The model under review builds one solid part; all positions refer to its coordinate system, in mm. A direction names the side the tool comes from. Coordinates: 2 decimals unless noted, no trailing zeros. Write each loop counter-clockwise with the first axis right and the second up, starting at its lowest first coordinate (ties: lowest second). Pieces come first, ordered by that corner, then holes. Notation, with made-up numbers: (-33.75, -22) - (7.25, -22) arc R24 cw to (7.25, -4) - close; hole circle Ø11 at (77.25, 18.5). An arc over 180 degrees is marked (long way). Return JSON: item names as keys, results as strings. Group by question number.
(1) Tool access review of faces 4 (the face through (-1.74, 6.11, 0.76)), 5 (the face through (-3, 2, 1.016)), 6 (the face through (-2, -5, 0.508)), 7 (the face through (1.75, 6.14, 0.76)): name each direction out of +Z, -Z, +X, -X, +Y, -Y from which nothing blocks a thin tool from reaching the whole face with its end or side.
(2) We need section B-B on x = 0. State the section outline as (y, z) points, then the cut area to 3 significant figures.
(3) To check wall thickness, follow L1, parallel to Y at x = 0, z = 0.1; L2, parallel to Z at x = -2.5, y = 3.5; L3, parallel to Z at x = -2, y = 5.5. State the ranges of each line that lie inside material, in increasing order. Write a range as from..to.
(4) Draft analysis for pull direction X (two halves, no side actions). For faces 1 (the face through (0, -7, 3.734)), 2 (the face through (1.75, -6.14, 0.76)), 3 (the face through (-0.75, -3.39, 0.25)), state which applies: released by +X, released by -X, zero draft, split by the parting line, or undercut.
(5) For pin 1 Ø2 at (x, z) = (-3, 0.5) entering from +Y; pin 2 Ø1.4 at (x, z) = (0.5, 2.5) entering from +Y; pin 3 Ø0.9 at (y, z) = (-7, 3) entering from +X, all flat-tipped, find the tip position at first contact; note any pin that passes through.
(6) We need section A-A on y = 0. State the section outline as (x, z) points, then the cut area to 3 significant figures.
(7) We need section C-C on z = 0.35. State the section outline as (x, y) points, then the cut area to 3 significant figures.
(8) We need section D-D on x = 4. State the section outline as (y, z) points, then the cut area to 3 significant figures.
```python
from build123d import *

# Parameters (mm, degrees)
SKETCH1_R           = 3.469974147
BOSS_EXTRUDE1_DEPTH = 0.508
BOSS_EXTRUDE2_DEPTH = 0.508
BOSS_EXTRUDE3_DEPTH = 2.7178
SKETCH4_R           = 3.429
BOSS_EXTRUDE4_DEPTH = 0.508


with BuildPart() as part:
    # Sketch1 → Boss-Extrude1 (new body)
    with BuildSketch(Plane.XY):
        with BuildLine():
            Line((-4.516012823, 6.325662964), (-4.516012823, -6.325662964))
            ThreePointArc((-4.516012823, -6.325662964), (0, -7.662131341), (4.516012823, -6.325662964))
            Line((4.516012823, -6.325662964), (4.516012823, 6.325662964))
            ThreePointArc((4.516012823, 6.325662964), (0, 7.662131341), (-4.516012823, 6.325662964))
        make_face()
        Circle(SKETCH1_R, mode=Mode.SUBTRACT)
    extrude(amount=BOSS_EXTRUDE1_DEPTH)

    # Sketch2 → Boss-Extrude2 (add)
    with BuildSketch(Plane.XY.offset(0.508)):
        with BuildLine():
            Line((2.209457086, -7.362582022), (1.281405607, -4.884037371))
            Line((1.281405607, -4.884037371), (-1.281405607, -4.884037371))
            Line((-1.281405607, -4.884037371), (-2.209457086, -7.362582022))
            ThreePointArc((-2.209457086, -7.362582022), (0, -7.662131341), (2.209457086, -7.362582022))
        make_face()
    boss_extrude2 = extrude(amount=BOSS_EXTRUDE2_DEPTH)

    # Sketch3 → Boss-Extrude3 (add)
    with BuildSketch(Plane.XY.offset(1.016)):
        with BuildLine():
            Line((-1.3716, -7.547991025), (-1.3716, -6.417691025))
            Line((-1.3716, -6.417691025), (1.3716, -6.417691025))
            Line((1.3716, -6.417691025), (1.3716, -7.547991025))
            ThreePointArc((1.3716, -7.547991025), (0, -7.662131341), (-1.3716, -7.547991025))
        make_face()
    extrude(amount=BOSS_EXTRUDE3_DEPTH)

    # Sketch4 → Boss-Extrude4 (add)
    with BuildSketch(Plane.XY.offset(0.508)):
        with BuildLine():
            Line((4.516012823, -1.692704651), (4.516012823, 1.692704651))
            ThreePointArc((4.516012823, 1.692704651), (0, 4.822822913), (-4.516012823, 1.692704651))
            Line((-4.516012823, 1.692704651), (-4.516012823, -1.692704651))
            ThreePointArc((-4.516012823, -1.692704651), (0, -4.822822913), (4.516012823, -1.692704651))
        make_face()
        Circle(SKETCH4_R, mode=Mode.SUBTRACT)
    extrude(amount=BOSS_EXTRUDE4_DEPTH)

    # Mirror1: Boss-Extrude2 across plane
    add(boss_extrude2.mirror(Plane.ZX))


solid = part.part
```
Ans:
{
 "1": {"face 4": "+Z, -X", "face 5": "+Z, +X, -X, +Y", "face 6": "+Z", "face 7": "+Z, +X"},
 "2": {"outline": "(-7.66, 0) - (-3.47, 0) - (-3.47, 0.51) - (-3.43, 0.51) - (-3.43, 1.02) - (-4.82, 1.02) - (-4.82, 0.51) - (-4.88, 0.51) - (-4.88, 1.02) - (-6.42, 1.02) - (-6.42, 3.73) - (-7.66, 3.73) - close; (3.43, 0.51) - (3.47, 0.51) - (3.47, 0) - (7.66, 0) - (7.66, 1.02) - (4.88, 1.02) - (4.88, 0.51) - (4.82, 0.51) - (4.82, 1.02) - (3.43, 1.02) - close", "area": "11.9 mm²"},
 "3": {"L1": "-7.66..-3.47, 3.47..7.66", "L2": "0..1.02", "L3": "0..0.51"},
 "4": {"face 1": "zero draft", "face 2": "released by +X", "face 3": "undercut"},
 "5": {"pin 1": "y = 7.42", "pin 2": "y = -6.42", "pin 3": "x = 1.37"},
 "6": {"outline": "(-4.52, 0) - (-3.47, 0) - (-3.47, 0.51) - (-3.43, 0.51) - (-3.43, 1.02) - (-4.52, 1.02) - close; (3.43, 0.51) - (3.47, 0.51) - (3.47, 0) - (4.52, 0) - (4.52, 1.02) - (3.43, 1.02) - close", "area": "2.17 mm²"},
 "7": {"outline": "(-4.52, -6.33) arc R8.3 ccw to (4.52, -6.33) - (4.52, 6.33) arc R8.3 ccw to (-4.52, 6.33) - close; hole circle Ø6.94 at (0, 0)", "area": "92.8 mm²"},
 "8": {"outline": "(-6.63, 0) - (6.63, 0) - (6.63, 0.51) - (2.69, 0.51) - (2.69, 1.02) - (-2.69, 1.02) - (-2.69, 0.51) - (-6.63, 0.51) - close", "area": "9.48 mm²"}
}
